Source: CAD feature listing. Evaluate the final solid. Frame: model axes, mm. A direction names the side the tool comes from. Round coordinates to 2 decimals unless told otherwise and drop trailing zeros. Write each loop counter-clockwise with the first axis right and the second up, starting at its lowest first coordinate (ties: lowest second). Pieces come first, ordered by that corner, then holes.
from build123d import *

# Parameters (mm, degrees)
F0_W        = 10
F0_H        = 4
F0_W_2      = 11
F1_DEPTH    = 5
F2_DEPTH    = 15
F4_DEPTH    = 40
F5_T1_DEPTH = 33.0017809158


# Not quite as in the source:
# - a fillet or chamfer that OpenCascade refuses, or shapes differently, is made with other operations: its cross-section is extruded or revolved along the edge and cut away or added


with BuildPart() as f1:
    # F0 (on Front) → F1 (new body)
    with BuildSketch(Plane.XZ):
        with Locations((0, 2)):
            Rectangle(F0_W, F0_H)
        with Locations((0, -2)):
            Rectangle(F0_W, F0_H)
        Polygon((16, -4), (5, -4), (-5, -4), (-16, -4), (-16, -7.5), (16, -7.5), align=None)
        Polygon((-5, 4), (5, 4), (16, 4), (20, 4), (20, 7.5), (-20, 7.5), (-20, 4), (-16, 4), align=None)
        with Locations((-10.5, -2)):
            Rectangle(F0_W_2, F0_H)
        with Locations((10.5, -2)):
            Rectangle(F0_W_2, F0_H)
        with Locations((10.5, 2)):
            Rectangle(F0_W_2, F0_H)
        with Locations((-10.5, 2)):
            Rectangle(F0_W_2, F0_H)
    extrude(amount=F1_DEPTH)

    # F0 (on Front) → F2 (join)
    with BuildSketch(Plane.XZ):
        Polygon((-5, 4), (5, 4), (16, 4), (20, 4), (20, 7.5), (-20, 7.5), (-20, 4), (-16, 4), align=None)
        with Locations((0, 2)):
            Rectangle(F0_W, F0_H)
        with Locations((0, -2)):
            Rectangle(F0_W, F0_H)
        Polygon((16, -4), (5, -4), (-5, -4), (-16, -4), (-16, -7.5), (16, -7.5), align=None)
    extrude(amount=F2_DEPTH)

    # F3 (on face) → F4 (cut)
    with BuildSketch(Plane.YZ.offset(20)):
        with BuildLine():
            ThreePointArc((-6.5, -5.75), (-6.7928932188, -5.0428932188), (-7.5, -4.75))
            Line((-7.5, -4.75), (-7.5, -6.75))
            ThreePointArc((-7.5, -6.75), (-6.7928932188, -6.4571067812), (-6.5, -5.75))
        make_face()
        with BuildLine():
            Line((-7.5, -6.75), (-7.5, -4.75))
            ThreePointArc((-7.5, -4.75), (-8.5, -5.75), (-7.5, -6.75))
        make_face()
        with BuildLine():
            ThreePointArc((-7.5, 6.75), (-8.5, 5.75), (-7.5, 4.75))
            Line((-7.5, 4.75), (-7.5, 6.75))
        make_face()
        with BuildLine():
            Line((-7.5, 6.75), (-7.5, 4.75))
            ThreePointArc((-7.5, 4.75), (-6.7928932188, 5.0428932188), (-6.5, 5.75))
            ThreePointArc((-6.5, 5.75), (-6.7928932188, 6.4571067812), (-7.5, 6.75))
        make_face()
    extrude(amount=-F4_DEPTH, mode=Mode.SUBTRACT)

    # F5: chamfer of 3.5 on 2 edges, made by hand

    # F5_s2 → F5_t1 (cut)
    with BuildSketch(Plane.XZ.offset(-9.0008904579)):
        Polygon((-12.5, -7.5), (-16, -4), (-16, -7.5), align=None)
        Polygon((16, -4), (12.5, -7.5), (16, -7.5), align=None)
    extrude(amount=F5_T1_DEPTH, mode=Mode.SUBTRACT)


solid = f1.part
1) Material intervals for line 1 (Z direction, x = 15, y = -11.75); line 2 (Z direction, x = 6, y = -11.5); line 3 (X direction, y = -4, z = 2.25), sorted ascending.
Taken from the geometry:
line 1: z = -5 to -4, 4 to 7.5
line 2: z = -7.5 to -4, 4 to 7.5
line 3: x = -16 to 16
2) Contact query for flat-ended pins moving along their axis: P1, Ø5, axis at x = -11, z = -0.5, coming from the -Y side; P2, Ø5.5, axis at y = -3, z = 0.5, coming from the +X side; P3, Ø4.5, axis at x = -15.5, y = -10, coming from the -Z side. Output: stop coordinate, or through.
Taken from the geometry:
P1: stops at y = -5
P2: stops at x = 16
P3: stops at z = -6.75
3) Section query B-B on z = 6.25. Return the cut outline in (x, y).
Taken from the geometry:
outline: (-20, -15) - (20, -15) - (20, -8.37) - (-20, -8.37) - close; (-20, -6.63) - (20, -6.63) - (20, 0) - (-20, 0) - close
4) Section query A-A on x = 0.5. Return the cut outline in (y, z), then the cut area to 3 significant figures.
Taken from the geometry:
outline: (-15, -7.5) - (0, -7.5) - (0, 7.5) - (-15, 7.5) - close; hole circle Ø2 at (-7.5, -5.75); hole circle Ø2 at (-7.5, 5.75)
area: 219 mm2
5) Section query C-C on y = -9.5. Return the cut outline in (x, z).
Taken from the geometry:
outline: (-20, 4) - (-5, 4) - (-5, -4) - (-16, -4) - (-12.5, -7.5) - (12.5, -7.5) - (16, -4) - (5, -4) - (5, 4) - (20, 4) - (20, 7.5) - (-20, 7.5) - close
6) Reachability of faces 1 (the face through (5, -10, 0)), 2 (the face through (-16, -2, 0)), 3 (the face through (-5, -10, 0)) from +Z, -Z, +X, -X, +Y, -Y: full face, straight path, thin tool, end or side. Return the list, or none.
Taken from the geometry:
face 1: +X, -Y
face 2: -Z, -X, +Y, -Y
face 3: -X, -Y
7) Section query D-D on x = -7.5. Return the cut outline in (y, z).
Taken from the geometry:
outline: (-15, -7.5) - (0, -7.5) - (0, 7.5) - (-15, 7.5) - (-15, 4) - (-5, 4) - (-5, -4) - (-15, -4) - close; hole circle Ø2 at (-7.5, -5.75); hole circle Ø2 at (-7.5, 5.75)
8) Pull-direction query (Z, two-part tool) for faces 4 (the face through (-13, -9, 4)), 5 (the face through (16, -2, 0)), 6 (the face through (-11, -5, 0)), 7 (the face through (15.4, -7.4, -4.6)); classes: released by +Z, released by -Z, zero draft, split by the parting line, or undercut.
Taken from the geometry:
face 4: undercut
face 5: zero draft
face 6: undercut
face 7: released by -Z
